For this review, use the dimensioned drawing (mm, ordinates from the lowest corner) and the shaded views. Coordinates: 2 decimals unless noted, no trailing zeros. Loops run counter-clockwise (first coordinate to the right, second up) from the corner with the lowest first, then second, coordinate; pieces in that order, holes last. Notation, with made-up numbers: (70, -32.75) - (104, -32.75) arc R20 ccw to (104, -25.75) - close; hole circle Ø10 at (26, 9.25). An arc over 180 degrees is marked (long way). Use one line per item in the form item = value. Start each with the question number.
(1) Add section C-C (y = 0.15). State the section outline as (x, z) points.
(2) Add section A-A (z = 35). State the section outline as (x, y) points, plus the area to 3 significant figures.
(3) For L1, parallel to X at y = 0.6, z = 35; L2, parallel to X at y = 0.4, z = 10, list the stretches that pass through material, from the lowest coordinate up.
(4) Add section D-D (z = 60). State the section outline as (x, y) points.
(5) Add section B-B (x = 35). State the section outline as (y, z) points, plus the area to 3 significant figures.
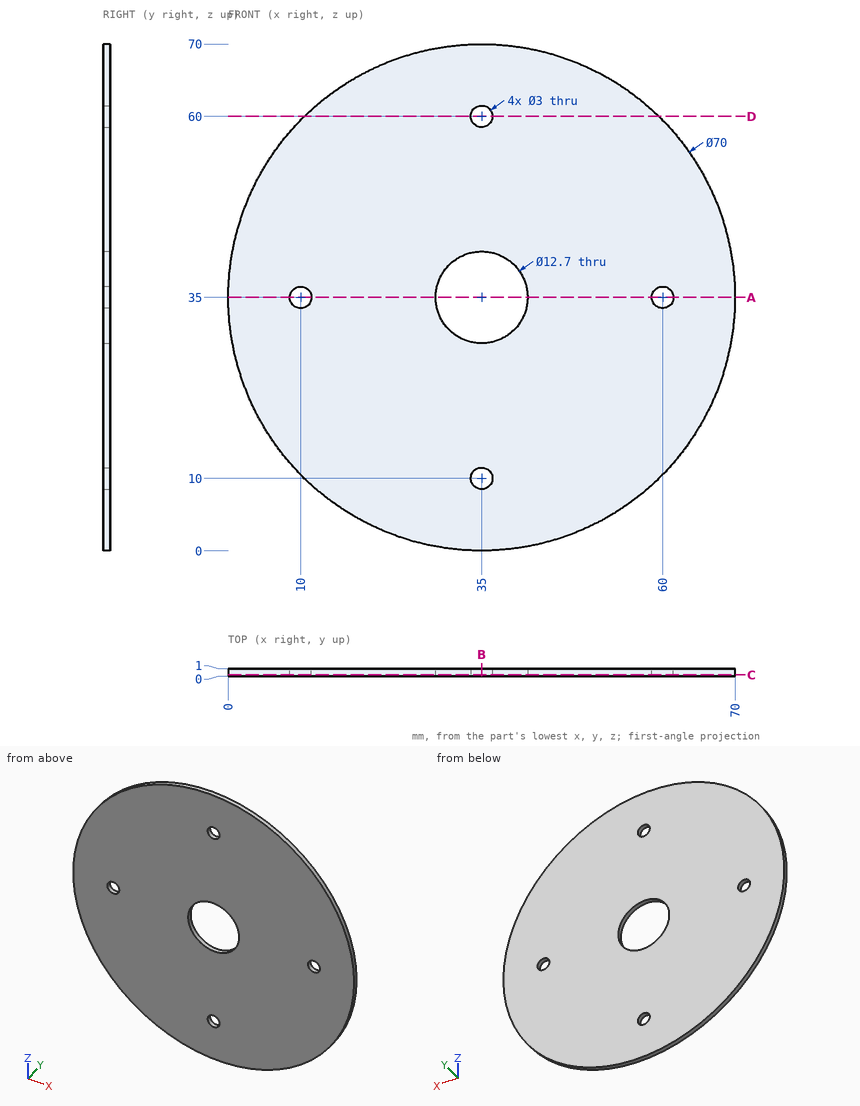
Computed values:
q1.outline = circle Ø70 at (35, 35); hole circle Ø3 at (10, 35); hole circle Ø12.7 at (35, 35); hole circle Ø3 at (35, 10); hole circle Ø3 at (35, 60); hole circle Ø3 at (60, 35)
q2.outline = (0, 0) - (8.5, 0) - (8.5, 1) - (0, 1) - close; (11.5, 0) - (28.65, 0) - (28.65, 1) - (11.5, 1) - close; (41.35, 0) - (58.5, 0) - (58.5, 1) - (41.35, 1) - close; (61.5, 0) - (70, 0) - (70, 1) - (61.5, 1) - close
q2.area = 51.3 mm^2
q3.L1 = 0 to 8.5, 11.5 to 28.65, 41.35 to 58.5, 61.5 to 70
q3.L2 = 10.51 to 33.5, 36.5 to 59.49
q4.outline = (10.51, 0) - (33.5, 0) - (33.5, 1) - (10.51, 1) - close; (36.5, 0) - (59.49, 0) - (59.49, 1) - (36.5, 1) - close
q5.outline = (0, 0) - (1, 0) - (1, 8.5) - (0, 8.5) - close; (0, 11.5) - (1, 11.5) - (1, 28.65) - (0, 28.65) - close; (0, 41.35) - (1, 41.35) - (1, 58.5) - (0, 58.5) - close; (0, 61.5) - (1, 61.5) - (1, 70) - (0, 70) - close
q5.area = 51.3 mm^2
